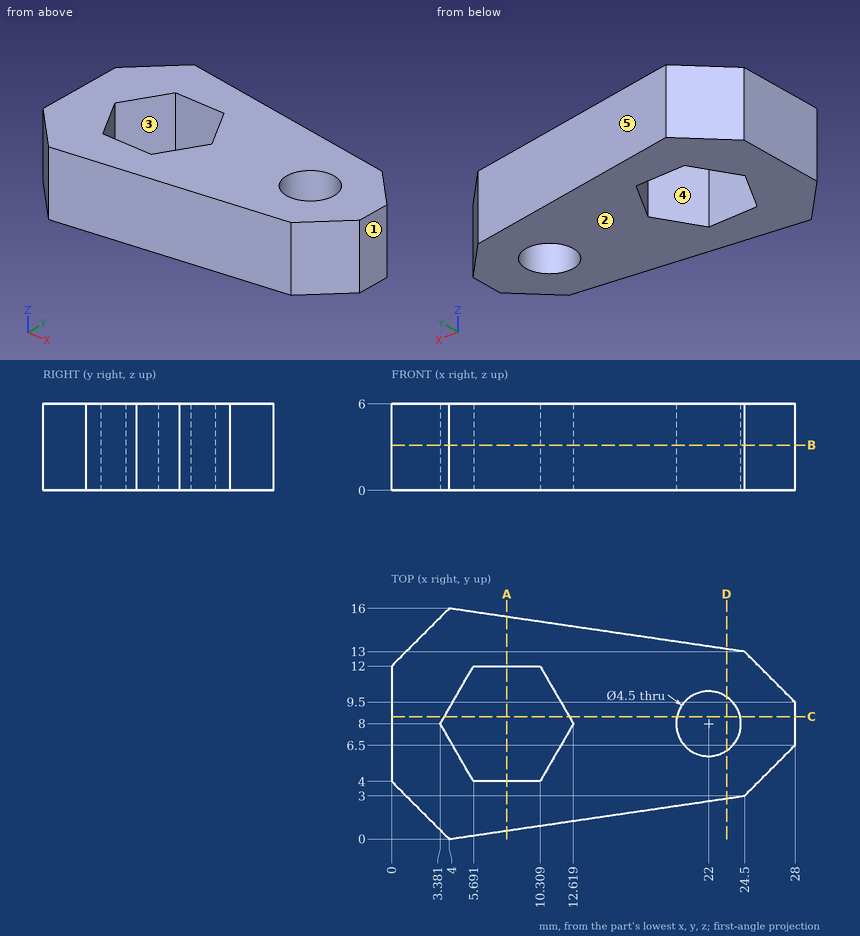
Input: dimensioned drawing with shaded views. Units: mm. Origin: part minimum x, y, z. A direction names the side the tool comes from. Round coordinates to 2 decimals unless told otherwise and drop trailing zeros. Order: outer loops, then holes, each group sorted by start corner. A loop starts at its lowest first (then second) coordinate and runs counter-clockwise, first axis right, second up. Notation, with made-up numbers: (-4.5, 7) -> (39.5, 7) arc R15 ccw to (39.5, 17) -> close; hole circle Ø3 at (33, 74.25). An arc over 180 degrees is marked (long way). One line per item, written item: value. Start each with the question number.
Q1. Material intervals for probe 1 along Y at (x, z) = (6.25, 0.35); probe 2 along X at (y, z) = (11.25, 4); probe 3 along Y at (x, z) = (22.5, 1.6), sorted ascending.
Q2. Access query for the marked faces 4 and 5. Directions: +Z, -Z, +X, -X, +Y, -Y. A direction counts if a zero-diameter tool reaches every point of the face in a straight line with its end or side. Return the directions, or none.
Q3. Section query C-C (y = 8.5). Return the cut outline in (x, z).
Q4. Pin query (flat end, axial travel): pin 1 (1.5 mm diameter, centred on x = 7, z = 1, fed in from -Y); pin 2 (2 mm diameter, centred on x = 9.5, z = 4, fed in from -Y); pin 3 (1.5 mm diameter, centred on y = 11, z = 1, fed in from +X). Return the tip coordinate at first contact, or that it passes through.
Q5. Draft query along X for the marked faces 1, 2 and 3. Return one class per face: pulls with the +X half, pulls with the -X half, needs draft (parallel to the pull), parting line crosses it, or undercut.
Q6. Section query A-A (x = 8). Return the cut outline in (y, z) (1 decimal).
Q7. Section query D-D (x = 23.25). Return the cut outline in (y, z).
Q8. Section query B-B (z = 3.15). Return the cut outline in (x, y).
Findings below:
1. probe 1: 0.33 to 4, 12 to 15.67
1. probe 2: 0 to 5.26, 10.74 to 26.25
1. probe 3: 2.71 to 5.81, 10.19 to 13.29
2. face 4: +Z, -Z
2. face 5: +Z, -Z, +X, +Y
3. outline: (0, 0) -> (3.67, 0) -> (3.67, 6) -> (0, 6) -> close; (12.33, 0) -> (19.81, 0) -> (19.81, 6) -> (12.33, 6) -> close; (24.19, 0) -> (28, 0) -> (28, 6) -> (24.19, 6) -> close
4. pin 1: y = 0.33
4. pin 2: y = 0.66
4. pin 3: x = 27.25
5. face 1: pulls with the +X half
5. face 2: needs draft
5. face 3: undercut
6. outline: (0.6, 0) -> (4, 0) -> (4, 6) -> (0.6, 6) -> close; (12, 0) -> (15.4, 0) -> (15.4, 6) -> (12, 6) -> close
7. outline: (2.82, 0) -> (6.13, 0) -> (6.13, 6) -> (2.82, 6) -> close; (9.87, 0) -> (13.18, 0) -> (13.18, 6) -> (9.87, 6) -> close
8. outline: (0, 4) -> (4, 0) -> (24.5, 3) -> (28, 6.5) -> (28, 9.5) -> (24.5, 13) -> (4, 16) -> (0, 12) -> close; hole (3.38, 8) -> (5.69, 4) -> (10.31, 4) -> (12.62, 8) -> (10.31, 12) -> (5.69, 12) -> close; hole circle Ø4.5 at (22, 8)
